Input: part model. Units: mm. Frame: model coordinates. A direction names the side the tool comes from. Give positions to 0.01 mm unless a question says otherwise; leave off trailing zeros. Order: outer loops, then holes, each group sorted by start corner. A loop starts at its lowest first (then second) coordinate and runs counter-clockwise, first axis right, second up. Notation, with made-up numbers: M 71,-28 L 128,-28 A16 cw 128,2 Z; hole C -34,-6 d11. An arc over 180 degrees is marked long. Use a Markdown table: item, result.
from build123d import *

# Parameters (mm, degrees)
SKETCH_1_W             = 16
SKETCH_1_H             = 16
EXTRUDE_1_DEPTH        = 80
SKETCH_2_R             = 6.5
CUT_EXTRUDE_1_DEPTH    = 50
SKETCH_10_W            = 12
SKETCH_10_H            = 8
SKETCH_10_H_2          = 3
CUT_EXTRUDE_2_DEPTH    = 10
SKETCH_11_R            = 3.25
CUT_EXTRUDE_5_DEPTH    = 1
HOLE_WIZARD_M4_1_D     = 3.3
HOLE_WIZARD_M4_1_DEPTH = 4
CUT_EXTRUDE_6_REACH    = 18
SKETCH_14_R            = 1
FILLET_1_R             = 1


with BuildPart() as part:
    # 草图1 → 凸台-拉伸1 (new body)
    with BuildSketch(Plane.XY):
        with Locations((8, -8)):
            Rectangle(SKETCH_1_W, SKETCH_1_H)
    extrude(amount=EXTRUDE_1_DEPTH)

    # 草图2 → 切除-拉伸1 (cut)
    with BuildSketch(Plane.XY.offset(80)):
        with Locations((8, -8)):
            Circle(SKETCH_2_R)
    extrude(amount=-CUT_EXTRUDE_1_DEPTH, mode=Mode.SUBTRACT)

    # 草图10 → 切除-拉伸2 (cut)
    with BuildSketch(Plane(origin=(0, 0, 0), x_dir=(-1, 0, 0), z_dir=(0, 0, -1))):
        with Locations((-8, -4)):
            Rectangle(SKETCH_10_W, SKETCH_10_H)
        with Locations((-8, -14.5)):
            Rectangle(SKETCH_10_W, SKETCH_10_H_2)
    extrude(amount=-CUT_EXTRUDE_2_DEPTH, mode=Mode.SUBTRACT)

    # 草图11 → 切除-拉伸5 (cut)
    with BuildSketch(Plane.XZ.offset(13)):
        with Locations((8, 5)):
            Circle(SKETCH_11_R)
    extrude(amount=-CUT_EXTRUDE_5_DEPTH, mode=Mode.SUBTRACT)

    # M4 螺纹孔的螺纹孔钻头1
    with Locations(Plane(origin=(0, -12, 0), x_dir=(-1, 0, 0), z_dir=(0, -1, 0))):
        with Locations((-8, -5)):
            Hole(HOLE_WIZARD_M4_1_D / 2, depth=HOLE_WIZARD_M4_1_DEPTH)

    # 草图14 → 切除-拉伸6 (cut, up to next)
    with BuildSketch(Plane(origin=(0, 0, 0), x_dir=(1, 0, 0), z_dir=(0, 1, 0)), mode=Mode.PRIVATE) as cut_extrude_6_sk1:
        with Locations((8, -40)):
            Circle(SKETCH_14_R)
    cut_extrude_6_tool1 = extrude(cut_extrude_6_sk1.sketch, amount=-CUT_EXTRUDE_6_REACH, mode=Mode.PRIVATE) & part.part
    add(cut_extrude_6_tool1.solids().sort_by_distance((8, 0, 40))[0], mode=Mode.SUBTRACT)

    # 圆角1
    fillet_1_edges = [part.edges().sort_by_distance(p)[0] for p in [
        (0, 0, 40),
        (16, 0, 40),
        (16, -16, 40),
        (0, -16, 40),
    ]]
    fillet(fillet_1_edges, radius=FILLET_1_R)


solid = part.part
1) Mould query, pull axis Z, two halves, no side actions, for faces 4 (the face through (1, -8, 80)), 5 (the face through (8, -4, 10)), 6 (the face through (2, -4, 5)), 7 (the face through (4.753, -12.507, 5.143)). Classes: released by +Z, released by -Z, zero draft, split by the parting line, or undercut.
Response values:
| item | result |
|---|---|
| face 4 | released by +Z |
| face 5 | released by -Z |
| face 6 | zero draft |
| face 7 | undercut |
2) Cut plane B-B on x = 8. Return loops of the section in (y, z).
Response values:
| item | result |
|---|---|
| outline | M -16,10 L -13,10 L -13,8.25 L -12,8.25 L -12,6.65 L -8,6.65 L -8,10 L 0,10 L 0,39 L -1.5,39 L -1.5,30 L -14.5,30 L -14.5,80 L -16,80 Z; M -13,0 L -8,0 L -8,3.35 L -12,3.35 L -12,1.75 L -13,1.75 Z; M -1.5,41 L 0,41 L 0,80 L -1.5,80 Z |
3) Material intervals for line 1 (X direction, y = -10.1, z = 5); line 2 (Y direction, x = 8, z = 53.5); line 3 (X direction, y = -1.05, z = 40), sorted ascending. Write a range as from..to.
Response values:
| item | result |
|---|---|
| line 1 | x = 0..6.35, 9.65..16 |
| line 2 | y = -16..-14.5, -1.5..0 |
| line 3 | x = 0..7, 9..16 |
4) Cut plane A-A on z = 5. Return loops of the section in (x, y), and give its area (3 significant figures).
Response values:
| item | result |
|---|---|
| outline | M 0,-15 A1 ccw 1,-16 L 2,-16 L 2,-13 L 4.75,-13 L 4.75,-12 L 6.35,-12 L 6.35,-8 L 2,-8 L 2,0 L 1,0 A1 ccw 0,-1 Z; M 9.65,-12 L 11.25,-12 L 11.25,-13 L 14,-13 L 14,-16 L 15,-16 A1 ccw 16,-15 L 16,-1 A1 ccw 15,0 L 14,0 L 14,-8 L 9.65,-8 Z |
| area | 103 mm² |
5) First-contact query: pin 1 Ø2 at (x, z) = (7.5, 6) entering from -Y; pin 2 Ø4 at (x, y) = (7, -7.5) entering from +Z; pin 3 Ø7.5 at (x, z) = (8, 5) entering from -Y; pin 4 Ø6.5 at (x, y) = (5, -4) entering from -Z. Flat tips, straight axial feed; report the tip coordinate or a pass-through.
Response values:
| item | result |
|---|---|
| pin 1 | stops at y = -12 |
| pin 2 | stops at z = 30 |
| pin 3 | stops at y = -13 |
| pin 4 | stops at z = 0 |
6) Cut plane C-C on z = 36. Return loops of the section in (x, y), and give its area (3 significant figures).
Response values:
| item | result |
|---|---|
| outline | M 0,-15 A1 ccw 1,-16 L 15,-16 A1 ccw 16,-15 L 16,-1 A1 ccw 15,0 L 1,0 A1 ccw 0,-1 Z; hole C 8,-8 d13 |
| area | 122 mm² |
7) Cut plane D-D on y = -10. Return loops of the section in (x, z).
Response values:
| item | result |
|---|---|
| outline | M 0,0 L 16,0 L 16,80 L 14.18,80 L 14.18,30 L 1.82,30 L 1.82,80 L 0,80 Z; hole C 8,5 d3.3 |
8) Reachability of faces 1 (the face through (10.999, -13.767, 55.35)), 2 (the face through (9.4, -8, 3.8)), 3 (the face through (9.4, -12, 3.6)) from +Z, -Z, +X, -X, +Y, -Y: full face, straight path, thin tool, end or side. Return the list, or none.
Response values:
| item | result |
|---|---|
| face 1 | +Z |
| face 2 | -Z, +Y |
| face 3 | -Y |
